Model file for the job. Use its own axes, mm. Coordinates: 2 decimals unless noted, no trailing zeros. Return JSON: item names as keys, results as strings. Group by question number.
1) Flat gauge pins, fed straight in: pin 1 (1.8 mm diameter, centred on x = 40, y = -70.35, fed in from +Z); pin 2 (1 mm diameter, centred on y = -16, z = 0.5, fed in from +X); pin 3 (4 mm diameter, centred on x = 80, y = -70.35, fed in from +Z). Where does each tip first touch, or does it go through?
2) Cut at A-A (z = 0.1). State how many separate pieces and enclosed holes the cut face has, and give its area (3 significant figures).
3) Probe line 1 (X direction, y = 37, z = -0.15); line 2 (Y direction, x = 0, z = 0.4); line 3 (X direction, y = -13, z = -0.2). List the from-to ranges inside material, lowest first.
from build123d import *

# Parameters (mm, degrees)
SKETCH_1_W          = 252.1
SKETCH_1_H          = 166.2
EXTRUDE_1_DEPTH     = 1
SKETCH_2_R          = 1.5
SKETCH_2_W          = 8.4
SKETCH_2_H          = 16.8
SKETCH_2_W_2        = 252.1
SKETCH_2_H_2        = 0.2
SKETCH_2_H_3        = 1
CUT_EXTRUDE1_DEPTH  = 10
SKETCH1_R           = 1.5
CUT_EXTRUDE2_DEPTH  = 10
SKETCH2_W           = 235.3
SKETCH2_H           = 8.1
BOSS_EXTRUDE1_DEPTH = 2


with BuildPart() as part:
    # 草图1 → 凸台-拉伸1 (new, symmetric)
    with BuildSketch(Plane.XY):
        Rectangle(SKETCH_1_W, SKETCH_1_H)
    extrude(amount=EXTRUDE_1_DEPTH, both=True)

    # 草图2 → Cut-Extrude1 (cut)
    with BuildSketch(Plane.XY.offset(1)):
        with Locations((-121.85, 73.3)):
            Circle(SKETCH_2_R)
        with Locations((-121.85, 37.3)):
            Circle(SKETCH_2_R)
        with Locations((-121.85, 1.3)):
            Circle(SKETCH_2_R)
        with Locations((-121.85, -34.7)):
            Circle(SKETCH_2_R)
        with Locations((-121.85, -70.7)):
            Circle(SKETCH_2_R)
        with Locations((121.85, -70.7)):
            Circle(SKETCH_2_R)
        with Locations((121.85, -34.7)):
            Circle(SKETCH_2_R)
        with Locations((121.85, 1.3)):
            Circle(SKETCH_2_R)
        with Locations((121.85, 37.3)):
            Circle(SKETCH_2_R)
        with Locations((121.85, 73.3)):
            Circle(SKETCH_2_R)
        with Locations((-121.85, 55.1)):
            Rectangle(SKETCH_2_W, SKETCH_2_H)
        with Locations((-121.85, 19.1)):
            Rectangle(SKETCH_2_W, SKETCH_2_H)
        with Locations((-121.85, -16.9)):
            Rectangle(SKETCH_2_W, SKETCH_2_H)
        with Locations((-121.85, -52.9)):
            Rectangle(SKETCH_2_W, SKETCH_2_H)
        with Locations((121.85, -52.9)):
            Rectangle(SKETCH_2_W, SKETCH_2_H)
        with Locations((121.85, -16.9)):
            Rectangle(SKETCH_2_W, SKETCH_2_H)
        with Locations((121.85, 19.1)):
            Rectangle(SKETCH_2_W, SKETCH_2_H)
        with Locations((121.85, 55.1)):
            Rectangle(SKETCH_2_W, SKETCH_2_H)
        with Locations((0, 83.089141708)):
            Rectangle(SKETCH_2_W_2, SKETCH_2_H_2)
        with Locations((0, -82.6)):
            Rectangle(SKETCH_2_W_2, SKETCH_2_H_3)
    extrude(amount=-CUT_EXTRUDE1_DEPTH, mode=Mode.SUBTRACT)

    # Sketch1 → Cut-Extrude2 (cut)
    with BuildSketch(Plane.XY.offset(1)):
        with Locations((100, -70.35)):
            Circle(SKETCH1_R)
        with Locations((80, -70.35)):
            Circle(SKETCH1_R)
        with Locations((60, -70.35)):
            Circle(SKETCH1_R)
        with Locations((40, -70.35)):
            Circle(SKETCH1_R)
        with Locations((20, -70.35)):
            Circle(SKETCH1_R)
        with Locations((0, -70.35)):
            Circle(SKETCH1_R)
        with Locations((-20, -70.35)):
            Circle(SKETCH1_R)
        with Locations((-40, -70.35)):
            Circle(SKETCH1_R)
        with Locations((-60, -70.35)):
            Circle(SKETCH1_R)
        with Locations((-80, -70.35)):
            Circle(SKETCH1_R)
        with Locations((-100, -70.35)):
            Circle(SKETCH1_R)
    extrude(amount=-CUT_EXTRUDE2_DEPTH, mode=Mode.SUBTRACT)

    # Sketch2 → Boss-Extrude1 (add)
    with BuildSketch(Plane.XY.offset(1)):
        with Locations((0, 87.039141708)):
            Rectangle(SKETCH2_W, SKETCH2_H)
    extrude(amount=-BOSS_EXTRUDE1_DEPTH)


solid = part.part
Answers below:
{
 "1": {"pin 1": "passes through", "pin 2": "stops at x = 117.65", "pin 3": "stops at z = 1"},
 "2": {"separate pieces": "1", "enclosed holes": "21", "area": "42,200 mm^2"},
 "3": {"line 1": "x = -126.05 to -123.32, -120.38 to 120.38, 123.32 to 126.05", "line 2": "y = -82.1 to -71.85, -68.85 to 91.09", "line 3": "x = -117.65 to 117.65"}
}
